Here's the drawing with two shaded views (mm, measured from the low corner). I have some questions. Give positions to 0.01 mm unless a question says otherwise; leave off trailing zeros. Loops run counter-clockwise (first coordinate to the right, second up) from the corner with the lowest first, then second, coordinate; pieces in that order, holes last.
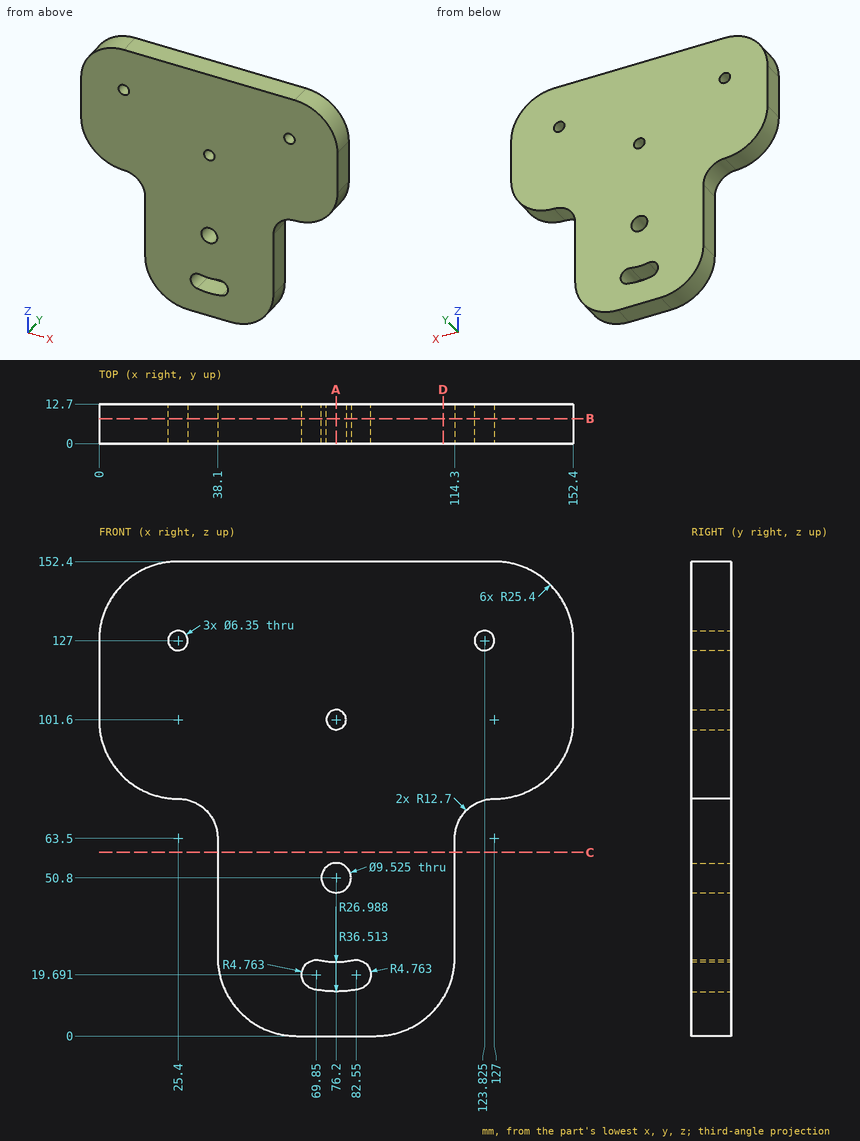
(1) Suppose I cut it at B-B on y = 8. Give the number of separate pieces and of enclosed holes in the cut face, plus the area to 3 significant figures.
Returned:
separate pieces: 1
enclosed holes: 5
area: 16,300 mm2
(2) Suppose I cut it at C-C on z = 59. List the corners of the cut face in (x, y) for me, plus the area to 3 significant figures.
Returned:
outline: (38.1, 0) - (114.3, 0) - (114.3, 12.7) - (38.1, 12.7) - close
area: 968 mm2
(3) Suppose I cut it at D-D on x = 110.5. List the corners of the cut face in (y, z) for me (1 decimal), plus the area to 3 significant figures.
Returned:
outline: (0, 12) - (12.7, 12) - (12.7, 152.4) - (0, 152.4) - close
area: 1,780 mm2
(4) Will these pins go through, and if not, where does the flat tip stop? P1, Ø2, axis at y = 6.5, z = 61.5, coming from the -X side; P2, Ø8.5, axis at x = 76.2, z = 50.8, coming from the +Y side; P3, Ø2, axis at x = 61, y = 6, coming from the -Z side.
Returned:
P1: stops at x = 38.1
P2: passes through
P3: stops at z = 0.04
(5) Suppose I cut it at A-A on x = 76.2. List the corners of the cut face in (y, z) for me (1 decimal).
Returned:
outline: (0, 0) - (12.7, 0) - (12.7, 14.3) - (0, 14.3) - close; (0, 23.8) - (12.7, 23.8) - (12.7, 46) - (0, 46) - close; (0, 55.6) - (12.7, 55.6) - (12.7, 98.4) - (0, 98.4) - close; (0, 104.8) - (12.7, 104.8) - (12.7, 152.4) - (0, 152.4) - close
(6) Please list where these lines run through material, in increasing order: probe 1 along Z at (x, y) = (76.2, 5.25) (1 decimal); probe 2 along X at (y, z) = (11, 58.5); probe 3 along Z at (x, y) = (23.5, 11.5) (1 decimal).
Returned:
probe 1: z = 0 to 14.3, 23.8 to 46, 55.6 to 98.4, 104.8 to 152.4
probe 2: x = 38.1 to 114.3
probe 3: z = 76.3 to 124.5, 129.5 to 152.3
